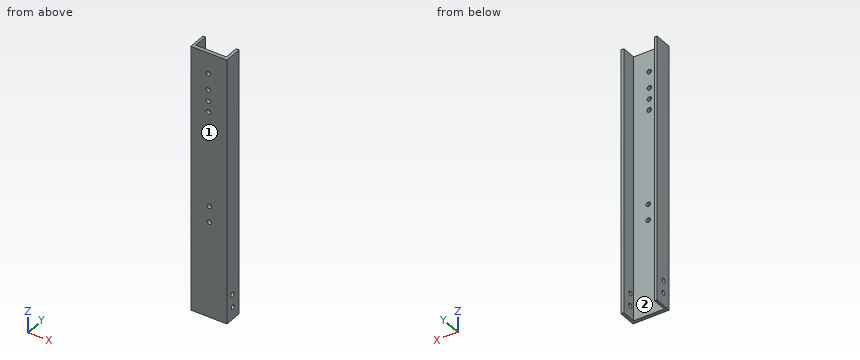
```python
from build123d import *

# Parameters (mm, degrees)
F0_W     = 25.4
F0_H     = 187.325
F1_DEPTH = 12.7
F2_W     = 21.59
F2_H     = 203.2
F3_DEPTH = 10.16
F5_D     = 3.175
F7_D     = 3.175
F9_D     = 3.175
F11_D    = 3.175
F13_D    = 3.175
F15_D    = 3.175
F17_D    = 3.175
F19_D    = 3.175


with BuildPart() as f1:
    # F0 (on Front) → F1 (new body)
    with BuildSketch(Plane.XZ):
        with Locations((-12.7, -39.635856)):
            Rectangle(F0_W, F0_H)
    extrude(amount=F1_DEPTH)

    # F2 (on Front) → F3 (cut)
    with BuildSketch(Plane.XZ):
        with Locations((-12.927838, -40.12759)):
            Rectangle(F2_W, F2_H)
    extrude(amount=F3_DEPTH, mode=Mode.SUBTRACT)

    # F5 (through all)
    with Locations(Plane.YZ):
        with Locations((-6.634117, -124.644481)):
            Hole(F5_D / 2)

    # F7 (through all)
    with Locations(Plane.YZ):
        with Locations((-6.922298, -115.689509)):
            Hole(F7_D / 2)

    # F9 (through all)
    with Locations(Plane(origin=(0, -10.16, 0), x_dir=(-1, 0, 0), z_dir=(0, 1, 0))):
        with Locations((13.036209, 39.331164)):
            Hole(F9_D / 2)

    # F11 (through all)
    with Locations(Plane(origin=(0, -10.16, 0), x_dir=(-1, 0, 0), z_dir=(0, 1, 0))):
        with Locations((13.172005, 27.753444)):
            Hole(F11_D / 2)

    # F13 (through all)
    with Locations(Plane(origin=(0, -10.16, 0), x_dir=(-1, 0, 0), z_dir=(0, 1, 0))):
        with Locations((13.182849, 19.840507)):
            Hole(F13_D / 2)

    # F15 (through all)
    with Locations(Plane(origin=(0, -10.16, 0), x_dir=(-1, 0, 0), z_dir=(0, 1, 0))):
        with Locations((13.062824, 12.179698)):
            Hole(F15_D / 2)

    # F17 (through all)
    with Locations(Plane(origin=(0, -10.16, 0), x_dir=(-1, 0, 0), z_dir=(0, 1, 0))):
        with Locations((12.404508, -54.598644)):
            Hole(F17_D / 2)

    # F19 (through all)
    with Locations(Plane(origin=(0, -10.16, 0), x_dir=(-1, 0, 0), z_dir=(0, 1, 0))):
        with Locations((12.404508, -65.762699)):
            Hole(F19_D / 2)


solid = f1.part
```
Geometry: final body of the model. Coordinates: model frame, mm. Face numbers are marked on the shaded views. Give positions to 0.01 mm unless a question says otherwise; leave off trailing zeros. Loops run counter-clockwise (first coordinate to the right, second up) from the corner with the lowest first, then second, coordinate; pieces in that order, holes last. Notation, with made-up numbers: (-4.75, 46) -> (45.25, 46) arc R9 ccw to (45.25, 58) -> close; hole circle Ø1 at (63.5, 16.25). An arc over 180 degrees is marked (long way). Use one line per item in the form item = value.
Item 1: Pin query (flat end, axial travel): P1, Ø2.5, axis at y = -6.63, z = -124.64, coming from the -X side; P2, Ø1.5, axis at x = -19, z = 27, coming from the +Y side. Return the tip coordinate at first contact, or that it passes through.
A:
P1 = through
P2 = -10.16
Item 2: Draft query along X for the marked faces 1 and 2. Return one class per face: pulls with the +X half, pulls with the -X half, needs draft (parallel to the pull), parting line crosses it, or undercut.
A:
face_1 = needs draft
face_2 = undercut
Item 3: Section query B-B on z = -87.5. Output: boundary loops of the cut face in (x, y), and give its area (3 significant figures).
A:
outline = (-25.4, -12.7) -> (0, -12.7) -> (0, 0) -> (-2.13, 0) -> (-2.13, -10.16) -> (-23.72, -10.16) -> (-23.72, 0) -> (-25.4, 0) -> close
area = 103 mm^2
Item 4: Line query: probe 1 along X at (y, z) = (-7.75, -68.5); probe 2 along Y at (x, z) = (-13.25, -44.5); probe 3 along X at (y, z) = (-10.5, 21). Output: solid intervals per line, ascending.
A:
probe_1 = -25.4 to -23.72, -2.13 to 0
probe_2 = -12.7 to -10.16
probe_3 = -25.4 to -14.27, -12.1 to 0
Item 5: Section query C-C on x = -7.5. Output: boundary loops of the cut face in (y, z).
A:
outline = (-12.7, -133.3) -> (-10.16, -133.3) -> (-10.16, 54.03) -> (-12.7, 54.03) -> close
Item 6: Section query A-A on y = -3.5. Output: boundary loops of the cut face in (x, z).
A:
outline = (-25.4, -133.3) -> (-23.72, -133.3) -> (-23.72, 54.03) -> (-25.4, 54.03) -> close; (-2.13, -133.3) -> (0, -133.3) -> (0, 54.03) -> (-2.13, 54.03) -> close
